Design review of the part built by this model. Coordinates are the model's own, in mm. A direction names the side the tool comes from. Give positions to 0.01 mm unless a question says otherwise; leave off trailing zeros. Write each loop counter-clockwise with the first axis right and the second up, starting at its lowest first coordinate (ties: lowest second). Pieces come first, ordered by that corner, then holes. Notation, with made-up numbers: (52.25, 82) - (95.25, 82) arc R27 ccw to (95.25, 109) - close; hole circle Ø1 at (-10, 28). An arc over 180 degrees is marked (long way). Use a Markdown table: item, result. Add a question column.
```python
from build123d import *

# Parameters (mm, degrees)
F0_R     = 6.35
F1_DEPTH = 31.75
F3_DEPTH = 31.751


with BuildPart() as f1:
    # F0 (on Front) → F1 (new body)
    with BuildSketch(Plane.XZ):
        with BuildLine():
            Line((53.7298298755, 11.3510093242), (-38.3451701245, 11.3510093242))
            ThreePointArc((-38.3451701245, 11.3510093242), (-54.2201701245, -4.5239906758), (-38.3451701245, -20.3989906758))
            Line((-38.3451701245, -20.3989906758), (53.7298298755, -20.3989906758))
            Line((53.7298298755, -20.3989906758), (53.6711269855, -10.9930955659))
            Line((53.6711269855, -10.9930955659), (12.3961269855, -10.9930955659))
            Line((12.3961269855, -10.9930955659), (12.3961269855, 1.7069044341))
            Line((12.3961269855, 1.7069044341), (53.6711269855, 1.7069044341))
            Line((53.6711269855, 1.7069044341), (53.7298298755, 11.3510093242))
        make_face()
        with Locations((-38.3451701245, -4.5239906758)):
            Circle(F0_R, mode=Mode.SUBTRACT)
    extrude(amount=F1_DEPTH)

    # F2 (on face) → F3 (cut, through all)
    with BuildSketch(Plane.XY.offset(11.3510093242)):
        with BuildLine():
            Line((53.7298298755, 0), (37.8548298755, 0))
            ThreePointArc((37.8548298755, 0), (49.0801500268, -4.6496798487), (53.7298298755, -15.875))
            Line((53.7298298755, -15.875), (53.7298298755, 0))
        make_face()
        with BuildLine():
            Line((53.7298298755, -31.75), (53.7298298755, -15.875))
            ThreePointArc((53.7298298755, -15.875), (49.0801500268, -27.1003201513), (37.8548298755, -31.75))
            Line((37.8548298755, -31.75), (53.7298298755, -31.75))
        make_face()
        Polygon((-38.3451701245, -22.2507314071), (-38.3451701245, -9.525), (-54.2339347303, -9.525), (-54.2339347303, -22.2551717675), align=None)
        Polygon((-12.9589347303, -9.525), (-38.3451701245, -9.525), (-38.3451701245, -22.2507314071), (-12.9589347303, -22.243636832), align=None)
        with BuildLine():
            ThreePointArc((37.8548298755, -22.225), (42.344957936, -20.3651280605), (44.2048298755, -15.875))
            ThreePointArc((44.2048298755, -15.875), (33.3647018149, -11.3848719395), (37.8548298755, -22.225))
        make_face()
    extrude(amount=-F3_DEPTH, mode=Mode.SUBTRACT)


solid = f1.part
```
(1) Insertion check: pin 1 (1 mm diameter, centred on x = -39.5, z = -10, fed in from +Y); pin 2 (10 mm diameter, centred on y = -7.5, z = -11, fed in from +X); pin 3 (6 mm diameter, centred on y = -16, z = -7, fed in from +X); pin 4 (6 mm diameter, centred on y = -17.5, z = -10, fed in from -X). Each pin has a flat end and moves straight along its axis. Give the tip position at first contact, or say it passes through.
(2) Add section A-A (y = -11). State the section outline as (x, z) points, and give its area (3 significant figures).
(3) Mouldability with a two-part tool opening along X and no side actions: class faces 4 (the face through (12.396, -16, -5)), 5 (the face through (8, -16, 11.351)), 6 (the face through (-32.48, -4.7, -6.96)) as +X half, -X half, draft (parallel to the pull), parting line (faces both ways), or undercut.
(4) Add section B-B (z = 3.5). State the section outline as (x, y) points (3 decimals), and give its area (3 significant figures).
(5) For line 1 along Y through (x, z) = (-13, 8) (3 decimals); line 2 along Y through (x, z) = (-37, -16) (3 decimals); line 3 along X through (y, z) = (-4.5, -4), list the stretches that pass through material, from the lowest coordinate up.
(6) Add section C-C (x = -16.5). State the section outline as (y, z) points (3 decimals), and give its area (3 significant figures).
(7) Add section D-D (z = -9). State the section outline as (x, y) points (3 decimals).
(8) Tool access review of faces 1 (the face through (-12.959, -16, -4)), 2 (the face through (29, -16, -10.993)), 3 (the face through (-54.216, -26.934, -4.175)): name each direction out of +Z, -Z, +X, -X, +Y, -Y from which nothing blocks a thin tool from reaching the whole face with its end or side.
Answers follow:
| question | item | result |
|---|---|---|
| 1 | pin 1 | through |
| 1 | pin 2 | x = 53.37 |
| 1 | pin 3 | x = 12.4 |
| 1 | pin 4 | x = -12.96 |
| 2 | outline | (-12.96, -20.4) - (33.79, -20.4) - (33.79, -10.99) - (12.4, -10.99) - (12.4, 1.71) - (33.79, 1.71) - (33.79, 11.35) - (-12.96, 11.35) - close; (41.92, -20.4) - (52.96, -20.4) - (52.96, -10.99) - (41.92, -10.99) - close; (41.92, 1.71) - (52.96, 1.71) - (52.96, 11.35) - (41.92, 11.35) - close |
| 2 | area | 1,420 mm^2 |
| 3 | face 4 | +X half |
| 3 | face 5 | draft |
| 3 | face 6 | undercut |
| 4 | outline | (-52.043, -31.75) - (37.855, -31.75) arc R15.875 ccw to (53.682, -17.106) - (53.682, -14.644) arc R15.875 ccw to (37.855, 0) - (-52.043, 0) - (-52.043, -9.525) - (-12.959, -9.525) - (-12.959, -22.244) - (-52.043, -22.255) - close; hole circle Ø12.7 at (37.855, -15.875) |
| 4 | area | 2,630 mm^2 |
| 5 | line 1 | -31.75 to -22.244, -9.525 to 0 |
| 5 | line 2 | -31.75 to -22.25, -9.525 to 0 |
| 5 | line 3 | -54.21 to -44.67, -32.02 to 12.4 |
| 6 | outline | (-31.75, -20.399) - (-22.245, -20.399) - (-22.245, 11.351) - (-31.75, 11.351) - close; (-9.525, -20.399) - (0, -20.399) - (0, 11.351) - (-9.525, 11.351) - close |
| 6 | area | 604 mm^2 |
| 7 | outline | (-53.576, -31.75) - (-42.849, -31.75) - (-42.849, -22.252) - (-53.576, -22.255) - close; (-53.576, -9.525) - (-42.849, -9.525) - (-42.849, 0) - (-53.576, 0) - close; (-33.841, -31.75) - (12.396, -31.75) - (12.396, 0) - (-33.841, 0) - (-33.841, -9.525) - (-12.959, -9.525) - (-12.959, -22.244) - (-33.841, -22.249) - close |
| 8 | face 1 | +Z, -Z, -X |
| 8 | face 2 | +X, +Y, -Y |
| 8 | face 3 | -X, +Y, -Y |
